Work out the finished part from the listing and answer in its coordinate system (mm). Face numbers are marked on the shaded views. A direction names the side the tool comes from. Round coordinates to 2 decimals unless told otherwise and drop trailing zeros. Order: outer loops, then holes, each group sorted by start corner. A loop starts at its lowest first (then second) coordinate and runs counter-clockwise, first axis right, second up. Notation, with made-up numbers: (22.25, -31) - (56.25, -31) arc R9 ccw to (56.25, -16) - close; hole circle Ø4 at (78.25, -21.75). An arc over 180 degrees is marked (long way). Use CSV: the item, a comma, the result in double quotes.
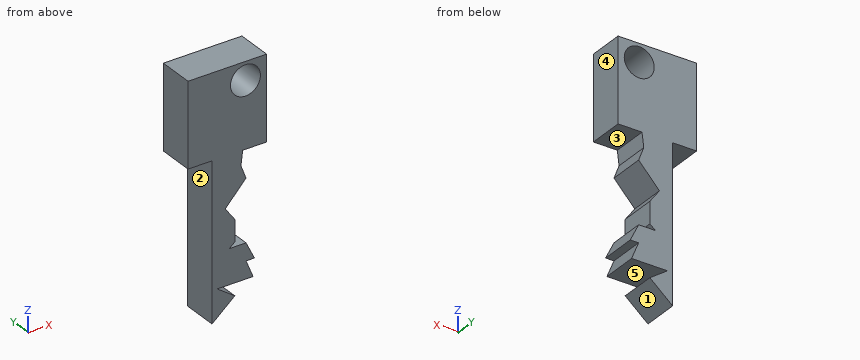
from build123d import *

# Parameters (mm, degrees)
F5_DEPTH = 3.81
F6_R     = 1.5875
F7_DEPTH = 25.4


# Not quite as in the source:
# - a feature of the source that left no trace in its solid (it failed there, or was rolled back) is left out


with BuildPart() as f5:
    # F3 (on offset) → F5 (new body)
    with BuildSketch(Plane.XZ.offset(25.4)):
        Polygon((15.9794489164, 25.4), (7.6507270483, 25.4), (7.6507270483, 16.51), (10.1907270483, 16.51), (10.1907270483, 0), (12.6087698864, 2.0575941857), (10.7351641334, 3.3673260217), (14.5451641334, 3.3673260217), (13.7953708033, 5.1956650805), (14.6843708033, 5.1956650805), (13.7953708033, 7.0228768909), (12.0173708033, 7.0228768909), (12.6087698864, 7.5033882066), (12.6087698864, 9.7893882066), (11.5895427104, 11.1838041431), (13.7953708033, 13.5722395859), (13.2549618376, 14.9972077083), (13.4394489164, 16.51), (15.9794489164, 16.51), align=None)
    extrude(amount=F5_DEPTH)

    # F6 (on face) → F7 (cut)
    with BuildSketch(Plane.XZ.offset(29.21)):
        with Locations((13.7358959764, 23.4795026481)):
            Circle(F6_R)
    extrude(amount=-F7_DEPTH, mode=Mode.SUBTRACT)


solid = f5.part
(1) The mould has two halves that part along Z. Classify the marked faces 1, 2 and 3: released by +Z, released by -Z, zero draft, split by the parting line, or undercut.
Findings below:
face 1,"released by -Z"
face 2,"zero draft"
face 3,"undercut"
(2) Find the intervals of material crossed by L1, parallel to Z at x = 13, y = -25.55; L2, parallel to Z at x = 8.5, y = -27.65; L3, parallel to Z at x = 11.75, y = -26.85, in increasing order. Write a range as from..to.
Findings below:
L1,"z = 3.37..7.02, 12.71..22.07, 24.89..25.4"
L2,"z = 16.51..25.4"
L3,"z = 1.33..2.66, 3.37..10.96, 11.36..25.4"
(3) For the marked faces 4 and 5, determine the directions among +Z, -Z, +X, -X, +Y, -Y from which every point of the face is accessible in a straight line to the end or side of a thin tool.
Findings below:
face 4,"+Z, -Z, +X, +Y, -Y"
face 5,"+X, +Y, -Y"
(4) Find section B-B (x = 9.5). Determine the outline of the cut face in (y, z).
Findings below:
outline,"(-29.21, 16.51) - (-25.4, 16.51) - (-25.4, 25.4) - (-29.21, 25.4) - close"
(5) Find section C-C (z = 9.5). Determine the outline of the cut face in (x, y).
Findings below:
outline,"(10.19, -29.21) - (12.61, -29.21) - (12.61, -25.4) - (10.19, -25.4) - close"
(6) Find section A-A (y = -25.7). Determine the outline of the cut face in (x, z) (1 decimal).
Findings below:
outline,"(7.7, 16.5) - (10.2, 16.5) - (10.2, 0) - (12.6, 2.1) - (10.7, 3.4) - (14.5, 3.4) - (13.8, 5.2) - (14.7, 5.2) - (13.8, 7) - (12, 7) - (12.6, 7.5) - (12.6, 9.8) - (11.6, 11.2) - (13.8, 13.6) - (13.3, 15) - (13.4, 16.5) - (16, 16.5) - (16, 25.4) - (7.7, 25.4) - close; hole circle Ø3.2 at (13.7, 23.5)"
(7) Each of these flat-tipped pins is pushed along its axis until it touches: pin 1 (2 mm diameter, centred on x = 9, y = -28, fed in from -Z); pin 2 (1 mm diameter, centred on x = 14, y = -27, fed in from -Z); pin 3 (1.1 mm diameter, centred on y = -26.5, z = 5.5, fed in from -X). Where does it stop, or does it pass through?
Findings below:
pin 1,"stops at z = 16.51"
pin 2,"stops at z = 3.37"
pin 3,"stops at x = 10.19"
